from build123d import *

# Parameters (mm, degrees)
SKETCH1_W           = 5
SKETCH1_H           = 30
SKETCH1_W_2         = 20
SKETCH1_H_2         = 5
BOSS_EXTRUDE1_DEPTH = 5


with BuildPart() as part:
    # Sketch1 → Boss-Extrude1 (new body)
    # profile 1 of 2: a face of its own
    with BuildSketch(Plane(origin=(0, 0, 0), x_dir=(1, 0, 0), z_dir=(0, 1, 0))):
        Polygon((69.5, -72), (69.5, 98), (61.25, 98), (-61.25, 98), (-69.5, 98), (-69.5, -72), (-45, -72), (-10, -72), (10, -72), (45, -72), align=None)
        with Locations((42.5, 0)):
            Rectangle(SKETCH1_W, SKETCH1_H, mode=Mode.SUBTRACT)
        with Locations((-42.5, 0)):
            Rectangle(SKETCH1_W, SKETCH1_H, mode=Mode.SUBTRACT)
    # profile 2 of 2: a face of its own
    with BuildSketch(Plane(origin=(0, 0, 0), x_dir=(1, 0, 0), z_dir=(0, 1, 0))):
        with Locations((0, -74.5)):
            Rectangle(SKETCH1_W_2, SKETCH1_H_2)
    extrude(amount=BOSS_EXTRUDE1_DEPTH)


solid = part.part
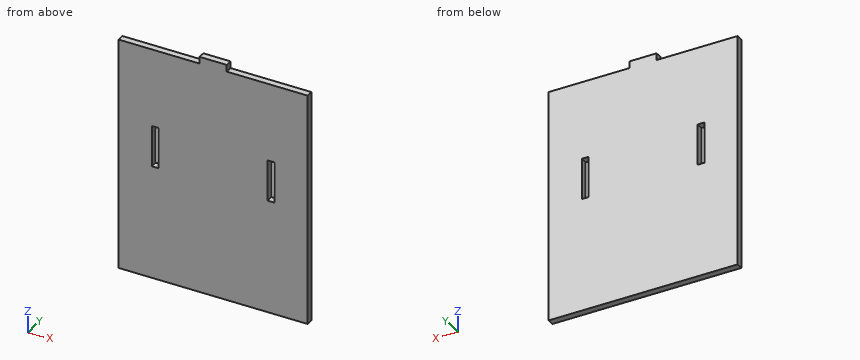
The listing builds one solid part. Answer for the finished solid, in the listing's coordinates (mm). Round coordinates to 2 decimals unless told otherwise and drop trailing zeros. Order: outer loops, then holes, each group sorted by start corner. A loop starts at its lowest first (then second) coordinate and runs counter-clockwise, first axis right, second up. Notation, with made-up numbers: (69, -19.75) - (109, -19.75) arc R25 ccw to (109, 7.25) - close; hole circle Ø1 at (61.5, 70.25). An arc over 180 degrees is marked (long way). Write item = value, one per line. Start each with the question number.
1) Straight lines are drawn through the part: L1, parallel to X at y = 3.85, z = -2; L2, parallel to Z at x = 43, y = 2.2; L3, parallel to Z at x = -23, y = 1.8. For each, find the intervals that lie inside material, in ascending order.
2) Section B-B, the plane y = 1.5 is taken. Write down the section's boundary in (x, z), plus the area to 3 significant figures.
3) Given pin 1 (1.5 mm diameter, centred on x = 42, y = 2, fed in from +Z), flat-ended and moving along its own axis, determine where the tip first touches the part or whether it passes through.
4) Section A-A, the plane z = 2 is taken. Write down the section's boundary in (x, y).
5) Section C-C, the plane x = 16.5 is taken. Write down the section's boundary in (y, z).
Results list:
q1.L1 = -69.5 to -45, -40 to 40, 45 to 69.5
q1.L2 = -98 to -15, 15 to 72
q1.L3 = -98 to 72
q2.outline = (-69.5, -98) - (69.5, -98) - (69.5, 72) - (10, 72) - (10, 77) - (-10, 77) - (-10, 72) - (-69.5, 72) - close; hole (-45, -15) - (-40, -15) - (-40, 15) - (-45, 15) - close; hole (40, -15) - (45, -15) - (45, 15) - (40, 15) - close
q2.area = 23,400 mm^2
q3.pin_1 = 72
q4.outline = (-69.5, 0) - (-45, 0) - (-45, 5) - (-69.5, 5) - close; (-40, 0) - (40, 0) - (40, 5) - (-40, 5) - close; (45, 0) - (69.5, 0) - (69.5, 5) - (45, 5) - close
q5.outline = (0, -98) - (5, -98) - (5, 72) - (0, 72) - close
